Verification items for the finished model (mm, model axes). Face numbers are marked on the shaded views. A direction names the side the tool comes from. Coordinates: 2 decimals unless noted, no trailing zeros. Order: outer loops, then holes, each group sorted by start corner. A loop starts at its lowest first (then second) coordinate and runs counter-clockwise, first axis right, second up. Notation, with made-up numbers: M -4,77.25 L 39,77.25 A11 cw 39,81.25 Z; hole C 23.25,-2.75 d8. An arc over 180 degrees is marked long. Write item = value, one per line.
Autodesk Inventor part; units mm, degrees
ref_plane "YZ Plane" through (0, 0, 0) normal (1, 0, 0) x (0, 1, 0)
ref_plane "XZ Plane" through (0, 0, 0) normal (0, 1, 0) x (-1, 0, 0)
ref_plane "XY Plane" through (0, 0, 0) normal (0, 0, 1) x (1, 0, 0)
sketch "Sketch1" plane through (0, 0, 0) normal (0, 0, 1) x (1, 0, 0)
  line L0 (0, 0) -> (0, 25.4)
  line L1 (0, 25.4) -> (9.1654, 41.275)
  line L2 (9.1654, 41.275) -> (18.3309, 25.4)
  line L3 (18.3309, 25.4) -> (24.6809, 25.4)
  line L4 (24.6809, 25.4) -> (33.8463, 41.275)
  line L5 (33.8463, 41.275) -> (43.0117, 25.4)
  line L6 (43.0117, 25.4) -> (83.9883, 25.4)
  line L7 (102.3191, 25.4) -> (108.6691, 25.4)
  line L8 (108.6691, 25.4) -> (117.8346, 41.275)
  line L9 (117.8346, 41.275) -> (127, 25.4)
  line L10 (127, 25.4) -> (127, 0)
  line L11 (127, 0) -> (88.9, 0)
  line L12 (88.9, 0) -> (104.775, -15.875)
  line L13 (104.775, -15.875) -> (22.225, -15.875)
  line L14 (22.225, -15.875) -> (38.1, 0)
  line L15 (38.1, 0) -> (0, 0)
  line L16 (9.1654, 41.275) -> (117.8346, 41.275) construction
  line L17 (102.3191, 25.4) -> (93.1537, 41.275)
  line L18 (83.9883, 25.4) -> (93.1537, 41.275)
  dimension "d0" = 45
  dimension "d1" = 45
  dimension "d2" = 127
  dimension "d3" = 60
  dimension "d4" = 6.35
  dimension "d5" = 25.4
  dimension "d6" = 25.4
  dimension "d7" = 38.1
  dimension "d8" = 15.875
  dimension "d9" = 6.35
  dimension "d10" = 60
  dimension "d12" = 60
  dimension "d13" = 25.4
  dimension "d14" = 25.4
  dimension "d15" = 25.4
  dimension "d16" = 15.875
  dimension "d17" = 60
extrude "MAIN BODY" add sketch "Sketch1" along normal mid plane 76.2
sketch "Sketch2" plane through (43.0117, 25.4, 38.1) normal (0, 1, 0) x (1, 0, 0)
  line L0 (7.7883, 12.7) -> (33.1883, 12.7)
  line L1 (33.1883, 12.7) -> (33.1883, 63.5)
  line L2 (33.1883, 63.5) -> (7.7883, 63.5)
  line L3 (7.7883, 63.5) -> (7.7883, 12.7)
  line L4 (40.9765, 0) -> (0, 0)
  line L5 (0, 76.2) -> (40.9765, 76.2)
  line L6 (40.9765, 76.2) -> (40.9765, 0)
  line L7 (0, 76.2) -> (0, 0)
  point P0 (-43.0117, 38.1)
  point P1 (20.4883, 12.7)
  dimension "d25" = 50.8
  dimension "d26" = 25.4
  dimension "d27" = 12.7
  dimension "d28" = 40.9765
  dimension "d29" = 7.7883
  dimension "d30" = 76.2
extrude "LARGE BOSS" add sketch "Sketch2" along normal blind 12.7 contours L3 L2 L1 L0
sketch "Sketch3" plane through (43.0117, 38.1, 38.1) normal (0, 1, 0) x (1, 0, 0)
  line L0 (7.7883, 12.7) -> (7.7883, 63.5)
  line L1 (9.2629, 38.1) -> (20.4883, 26.8747)
  line L2 (20.4883, 26.8747) -> (31.7136, 38.1)
  line L3 (31.7136, 38.1) -> (20.4883, 49.3253)
  line L4 (20.4883, 49.3253) -> (9.2629, 38.1)
  line L5 (33.1883, 12.7) -> (33.1883, 63.5)
  line L6 (7.7883, 63.5) -> (33.1883, 63.5)
  line L7 (20.4883, 63.5) -> (20.4883, 12.7) construction
  line L8 (7.7883, 12.7) -> (33.1883, 12.7)
  line L9 (7.7883, 38.1) -> (33.1883, 38.1) construction
  point P0 (-43.0117, 38.1)
  dimension "d34" = 15.875
  dimension "d35" = 15.875
  dimension "d36" = 45
extrude "TALL BOSS" add sketch "Sketch3" along normal blind 25.4 contours L4 L3 L2 L1
sketch "Sketch4" plane through (43.0117, 63.5, 38.1) normal (0, 1, 0) x (1, 0, 0)
  line L0 (20.4883, 49.3253) -> (9.2629, 38.1)
  line L1 (20.4883, 26.8747) -> (31.7136, 38.1)
  line L2 (9.2629, 38.1) -> (31.7136, 38.1)
  line L3 (31.7136, 38.1) -> (20.4883, 49.3253)
  line L4 (20.4883, 49.3253) -> (20.4883, 26.8747)
  point P0 (-43.0117, 38.1)
  point P1 (20.4883, 38.1)
hole "THROUGH HOLE" at (63.5, 63.5, 0) direction (0, -1, 0) diameter 9.525 end through all
fillet "LARGE BOSS FILLET" radius 6.35 4 edges at (76.2, 25.4, 0) (63.5, 25.4, -25.4) (50.8, 25.4, 0) (63.5, 25.4, 25.4)
equation "\"d1\" = d0"
equation "\"d6\" = d5"
equation "\"d9\" = d4"
equation "\"d10\" = d3"
equation "\"d12\" = d11"
equation "\"d13\" = d6"
equation "\"d14\" = d13"
equation "\"d29\" = -0.5 * d26 + 0.5 * d28"
equation "\"d11\" = d10"
properties part number "2020-10-BK" material "Gold"
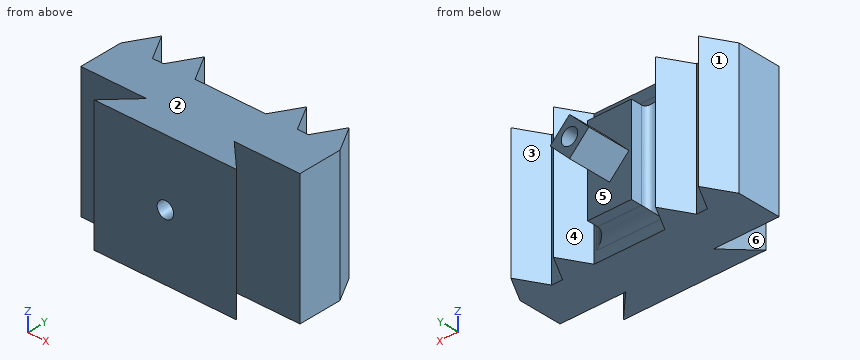
Item 1: Release check for a two-part mould opening along X. For the marked faces 1, 2 and 3 record: pulls with the +X half, pulls with the -X half, needs draft (parallel to the pull), parting line crosses it, or undercut.
Report:
face_1 = pulls with the -X half
face_2 = needs draft
face_3 = undercut
Item 2: Sectioned sample at C-C, the plane z = -22.5. Enter the section's corners in (x, y) (3 decimals), then the cut area to 3 significant figures.
Report:
outline = M 0,0 L 38.1,0 L 22.225,-15.875 L 104.775,-15.875 L 88.9,0 L 127,0 L 127,25.4 L 117.835,41.275 L 108.669,25.4 L 102.319,25.4 L 93.154,41.275 L 83.988,25.4 L 82.55,25.4 A6.35 cw 76.2,31.75 L 76.2,38.1 L 50.8,38.1 L 50.8,31.75 A6.35 cw 44.45,25.4 L 43.012,25.4 L 33.846,41.275 L 24.681,25.4 L 18.331,25.4 L 9.165,41.275 L 0,25.4 Z
area = 5,210 mm^2
Item 3: Gauge pin test, flat ends, axial feed: pin 1 (3 mm diameter, centred on y = 36, z = -5.5, fed in from +X); pin 2 (11.5 mm diameter, centred on x = 115.5, z = 4, fed in from -Y); pin 3 (5 mm diameter, centred on x = 106.5, z = 12, fed in from +Y). Record the tip position at first contact, or that the pin passes through.
Report:
pin_1 = 121.75
pin_2 = 0
pin_3 = 25.97
Item 4: Scan lines: L1, parallel to X at y = 46, z = 0; L2, parallel to Z at x = 63, y = 24; L3, parallel to Z at x = 63.5, y = 1.5. Record each from-to range of solid material in increasing order. Write a range as from..to.
Report:
L1 = 52.27..58.74, 68.26..74.73
L2 = -38.1..-4.74, 4.74..38.1
L3 = -38.1..-4.76, 4.76..38.1
Item 5: Tool access check on the marked faces 4, 5 and 6. Record the directions out of +Z, -Z, +X, -X, +Y, -Y that give a thin tool (end or side, any length) a straight path to the whole face; none if there is none.
Report:
face_4 = +Z, -Z, +Y
face_5 = +Y
face_6 = +Z, -Z, -X
Item 6: Sectioned sample at B-B, the plane y = 51. Enter the section's corners in (x, z) (1 decimal), then the cut area to 3 significant figures.
Report:
outline = M 52.3,0 L 63.5,-11.2 L 74.7,0 L 63.5,11.2 Z; hole C 63.5,0 d9.5
area = 181 mm^2
Item 7: Sectioned sample at D-D, the plane x = 54.5. Enter the section's corners in (y, z) (3 decimals), then the cut area to 3 significant figures.
Report:
outline = M -15.875,-38.1 L 25.4,-38.1 L 25.4,-31.75 A6.35 cw 31.75,-25.4 L 38.1,-25.4 L 38.1,-2.225 L 63.5,-2.225 L 63.5,2.225 L 38.1,2.225 L 38.1,25.4 L 31.75,25.4 A6.35 cw 25.4,31.75 L 25.4,38.1 L -15.875,38.1 Z
area = 3,920 mm^2
Item 8: Sectioned sample at A-A, the plane y = 27. Enter the section's corners in (x, z) (1 decimal).
Report:
outline = M 0.9,-38.1 L 17.4,-38.1 L 17.4,38.1 L 0.9,38.1 Z; M 25.6,-38.1 L 42.1,-38.1 L 42.1,38.1 L 25.6,38.1 Z; M 48.7,-27.5 L 78.3,-27.5 L 78.3,27.5 L 48.7,27.5 Z; M 84.9,-38.1 L 101.4,-38.1 L 101.4,38.1 L 84.9,38.1 Z; M 109.6,-38.1 L 126.1,-38.1 L 126.1,38.1 L 109.6,38.1 Z; hole C 63.5,0 d9.5
